Source: CAD feature listing. Evaluate the final solid. Frame: model axes, mm. Face numbers are marked on the shaded views. A direction names the side the tool comes from. Coordinates: 2 decimals unless noted, no trailing zeros. Write each loop counter-clockwise with the first axis right and the second up, starting at its lowest first coordinate (ties: lowest second). Pieces come first, ordered by that corner, then holes. Notation, with made-up numbers: (73, 73.25) - (99, 73.25) arc R27 cw to (99, 95.25) - close; hole circle Ø4 at (44.25, 31). An arc over 180 degrees is marked (long way). One line per question, with ' | ' between items.
from build123d import *

# Parameters (mm, degrees)
BOSS_EXTRUDE1_DEPTH = 7.5
FILLET1_R           = 6
FILLET2_R           = 4
BOSS_EXTRUDE2_DEPTH = 15
LPATTERN1_COUNT     = 6
LPATTERN1_PITCH     = 6
CUT_EXTRUDE1_DEPTH  = 26
CUT_EXTRUDE2_DEPTH  = 5
SKETCH5_R           = 1.5
CUT_EXTRUDE3_DEPTH  = 130.931165931
SKETCH6_R           = 1.75
BOSS_EXTRUDE3_DEPTH = 3
SKETCH7_R           = 1.25
CUT_EXTRUDE4_DEPTH  = 1
SKETCH8_R           = 1.25
CUT_EXTRUDE5_DEPTH  = 1
CUT_EXTRUDE6_DEPTH  = 1


with BuildPart() as part:
    # Sketch1 → Boss-Extrude1 (new, symmetric)
    with BuildSketch(Plane(origin=(0, 0, 0), x_dir=(0, 1, 0), z_dir=(0, 0, 1))):
        with BuildLine():
            Line((-12.93657624, 0), (-36.683093305, -3.478926169))
            Line((-36.683093305, -3.478926169), (-15.74375395, -70.273716889))
            Line((-15.74375395, -70.273716889), (-17.80717771, -70.273716889))
            Line((-17.80717771, -70.273716889), (-21.696997284, -79.486170616))
            Line((-21.696997284, -79.486170616), (-12.467013439, -88.640808687))
            Line((-12.467013439, -88.640808687), (-3.493010858, -117.267147567))
            Line((-3.493010858, -117.267147567), (-3.493010858, -124.267147567))
            Line((-3.493010858, -124.267147567), (6.506989142, -124.267147567))
            Line((6.506989142, -124.267147567), (6.506989142, -74.267147567))
            Line((6.506989142, -74.267147567), (12.638392495, -66.367407513))
            ThreePointArc((12.638392495, -66.367407513), (10.129821893, -59.756274968), (3.518689347, -62.26484557))
            Line((3.518689347, -62.26484557), (2.19282229, -70.273716889))
            Line((2.19282229, -70.273716889), (-2.80717771, -70.273716889))
            Line((-2.80717771, -70.273716889), (-12.93657624, 0))
        make_face()
    extrude(amount=BOSS_EXTRUDE1_DEPTH, both=True)

    # Fillet1
    fillet1_edges = [part.edges().sort_by_distance(p)[0] for p in [
        (3.478926169, -36.683093305, 0),
        (0, -12.93657624, 0),
    ]]
    fillet(fillet1_edges, radius=FILLET1_R)

    # Fillet2
    # the kernel refuses this fillet: 4 mm, written as the material it takes off along each edge
    with BuildSketch(Plane(origin=(124.267147567, -3.493010858, -17.5), x_dir=(0, 1, 0), z_dir=(0, 0, 1))) as fillet2_piece_1:
        with BuildLine():
            CenterArc((FILLET2_R, FILLET2_R), FILLET2_R, 180, 90)
            Line((0, FILLET2_R), (-FILLET2_R * 0.02, FILLET2_R))
            Line((-FILLET2_R * 0.02, FILLET2_R), (-FILLET2_R * 0.02, -FILLET2_R * 0.02))
            Line((-FILLET2_R * 0.02, -FILLET2_R * 0.02), (FILLET2_R, -FILLET2_R * 0.02))
            Line((FILLET2_R, -FILLET2_R * 0.02), (FILLET2_R, 0))
        make_face()
    extrude(amount=35, mode=Mode.SUBTRACT)
    with BuildSketch(Plane(origin=(70.273716889, -17.80717771, -14.005853421), x_dir=(0, 1, 0), z_dir=(0, 0, 1))) as fillet2_piece_2_section:
        with BuildLine():
            CenterArc((2.672717651, -3.953322774), FILLET2_R, 98.761599305, 58.347232051)
            Line((-1.012263839, -2.397394944), (-1.085963469, -2.366276387))
            Line((-1.085963469, -2.366276387), (-0.07369963, 0.031118557))
            Line((-0.07369963, 0.031118557), (0, 0.08))
            ThreePointArc((0, 0.08), (1.03171188, 0.08), (2.051237882, 0.079066455))
            Line((2.051237882, 0.079066455), (2.06342376, 0))
        make_face()
    fillet2_piece_2 = extrude(amount=28.011706842, mode=Mode.PRIVATE)
    fillet2_piece_2 = split(fillet2_piece_2, bisect_by=Plane(origin=(70.257081216, -15.748969027, 0), z_dir=(0.2991334193615799, -0.954211296003694, 0)), keep=Keep.TOP, mode=Mode.PRIVATE)
    add(fillet2_piece_2, mode=Mode.SUBTRACT)
    with BuildSketch(Plane(origin=(79.486170616, -21.696997284, -14.26109301), x_dir=(-0.9212453727262618, 0.3889819574613337, 0), z_dir=(0, 0, 1))) as fillet2_piece_3:
        with BuildLine():
            CenterArc((FILLET2_R * 0.676109301023, -FILLET2_R), FILLET2_R, 90, 68.125982867)
            Line((-FILLET2_R * 0.251896002422, -FILLET2_R * 0.627433017057), (-FILLET2_R * 0.270456108491, -FILLET2_R * 0.619981677398))
            Line((-FILLET2_R * 0.270456108491, -FILLET2_R * 0.619981677398), (-FILLET2_R * 0.0135221860205, FILLET2_R * 0.02))
            Line((-FILLET2_R * 0.0135221860205, FILLET2_R * 0.02), (FILLET2_R * 0.676109301023, FILLET2_R * 0.02))
            Line((FILLET2_R * 0.676109301023, FILLET2_R * 0.02), (FILLET2_R * 0.676109301023, 0))
        make_face()
    extrude(amount=28.52218602, mode=Mode.SUBTRACT)

    # Sketch2 → Boss-Extrude2 (add)
    with BuildSketch(Plane.XY.offset(7.5)):
        Polygon((119.267147567, 6.506989142), (121.267147567, 6.506989142), (119.267147567, 10.506989142), align=None)
        Polygon((117.267147567, 6.506989142), (119.267147567, 6.506989142), (119.267147567, 10.506989142), align=None)
    boss_extrude2 = extrude(amount=-BOSS_EXTRUDE2_DEPTH)

    # LPattern1: Boss-Extrude2 ×6
    with Locations(*[(-i * LPATTERN1_PITCH, 0, 0) for i in range(1, LPATTERN1_COUNT)]):
        add(boss_extrude2)

    # Sketch3 → Cut-Extrude1 (cut)
    with BuildSketch(Plane.XY.offset(7.5)):
        Polygon((118.41479062, 4.13462657), (86.532799982, 3.176685284), (86.532799982, -9.820815038), (116.995150337, -0.75112261), align=None)
    extrude(amount=-CUT_EXTRUDE1_DEPTH, mode=Mode.SUBTRACT)

    # Sketch4 → Cut-Extrude2 (cut)
    with BuildSketch(Plane(origin=(11.490191231, -36.652776175, 0), x_dir=(0.954211296003694, 0.2991334193615799, 0), z_dir=(0.29913341936157983, -0.9542112960036939, 0))):
        Polygon((85.852760577, 3.5), (85.852760577, -3.5), (106.852760577, -0.5), (106.852760577, 0.5), align=None)
    extrude(amount=-CUT_EXTRUDE2_DEPTH, mode=Mode.SUBTRACT)

    # Sketch5 → Cut-Extrude3 (cut, through all)
    with BuildSketch(Plane.XY.offset(7.5)):
        with Locations((8.395954367, -28.853750382)):
            Circle(SKETCH5_R)
    extrude(amount=-CUT_EXTRUDE3_DEPTH, mode=Mode.SUBTRACT)

    # Sketch6 → Boss-Extrude3 (add)
    with BuildSketch(Plane.XY.offset(7.5)):
        with Locations(Location((78.550648186, -16.960038516, 0), (0, 0, 180))):
            Circle(SKETCH6_R)
        with Locations(Location((64.316126541, 8.078540921, 0), (0, 0, 180))):
            Circle(SKETCH6_R)
    boss_extrude3 = extrude(amount=BOSS_EXTRUDE3_DEPTH)

    # Sketch7 → Cut-Extrude4 (cut)
    with BuildSketch(Plane.XY.offset(10.5)):
        with Locations((78.550648186, -16.960038516)):
            Circle(SKETCH7_R)
    cut_extrude4 = extrude(amount=-CUT_EXTRUDE4_DEPTH, mode=Mode.SUBTRACT)

    # Sketch8 → Cut-Extrude5 (cut)
    with BuildSketch(Plane.XY.offset(10.5)):
        with Locations((64.316126541, 8.078540921)):
            Circle(SKETCH8_R)
    cut_extrude5 = extrude(amount=-CUT_EXTRUDE5_DEPTH, mode=Mode.SUBTRACT)

    # Sketch9 → Cut-Extrude6 (cut)
    with BuildSketch(Plane.XY.offset(7.5)):
        with BuildLine():
            Line((15.753388713, -22.103953925), (62.646298586, -10.0457771))
            ThreePointArc((62.646298586, -10.0457771), (65.390728962, -11.667485959), (63.769020103, -14.411916335))
            Line((63.769020103, -14.411916335), (16.87611023, -26.470093159))
            ThreePointArc((16.87611023, -26.470093159), (14.131679854, -24.848384301), (15.753388713, -22.103953925))
        make_face()
    cut_extrude6 = extrude(amount=-CUT_EXTRUDE6_DEPTH, mode=Mode.SUBTRACT)

    # Mirror1: Boss-Extrude3, Cut-Extrude4, Cut-Extrude5, Cut-Extrude6 across plane
    add(boss_extrude3.mirror(Plane.XY))
    add(cut_extrude4.mirror(Plane.XY), mode=Mode.SUBTRACT)
    add(cut_extrude5.mirror(Plane.XY), mode=Mode.SUBTRACT)
    add(cut_extrude6.mirror(Plane.XY), mode=Mode.SUBTRACT)


solid = part.part
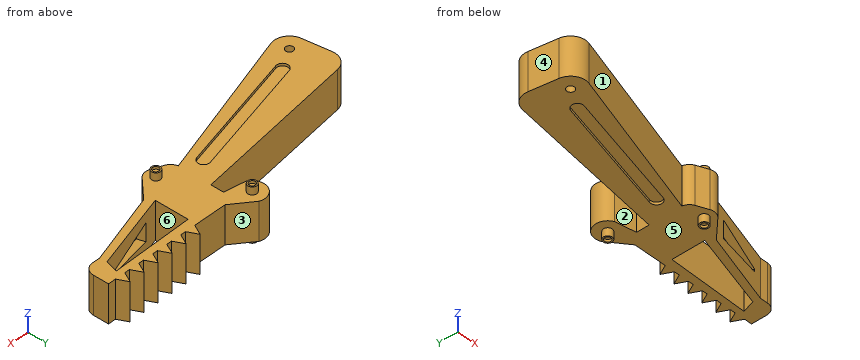
Item 1: Cut plane C-C on z = -4.75. State how many separate pieces and enclosed holes the cut face has, and give its area (3 significant figures).
Check sheet entries:
separate pieces: 1 | enclosed holes: 2 | area: 2,070 mm²
Item 2: Pin query (flat end, axial travel): pin 1 Ø5 at (x, z) = (14.5, -7.5) entering from +Y; pin 2 Ø3 at (x, z) = (24, -6) entering from -Y; pin 3 Ø2 at (x, y) = (55.5, -21.5) entering from +Z; pin 4 Ø2 at (x, y) = (21.5, -26) entering from +Z. Return the tip coordinate at first contact, or that it passes through.
Check sheet entries:
pin 1: y = -10.49 | pin 2: y = -30.72 | pin 3: through | pin 4: z = 7.5
Item 3: Cut plane D-D on x = 22. Return loops of the section in (y, z), and give its area (3 significant figures).
Check sheet entries:
outline: (-30.88, -7.5) - (-25.15, -7.5) - (-25.15, -6.5) - (-20.5, -6.5) - (-20.5, -7.5) - (-9.77, -7.5) - (-9.77, 7.5) - (-20.5, 7.5) - (-20.5, 6.5) - (-25.15, 6.5) - (-25.15, 7.5) - (-30.88, 7.5) - close | area: 307 mm²
Item 4: Ray query, line 1 along Z through (x, y) = (27.5, -22); line 2 along Z through (x, y) = (58, -7); line 3 along Y through (x, z) = (63, 3). Return the intervals inside material, ascending. Write a range as [from, to].
Check sheet entries:
line 1: [-6.5, 6.5] | line 2: [-7.5, 7.5] | line 3: [-18.02, -3.86], [3.4, 12.9]
Item 5: Mould query, pull axis X, two halves, no side actions, for the marked faces 4, 5 and 6. Classes: pulls with the +X half, pulls with the -X half, needs draft (parallel to the pull), parting line crosses it, or undercut.
Check sheet entries:
face 4: pulls with the -X half | face 5: needs draft | face 6: undercut
Item 6: Cut plane A-A on x = 68.5. Return loops of the section in (y, z).
Check sheet entries:
outline: (-16.3, -7.5) - (-3.06, -7.5) - (-3.06, 7.5) - (-16.3, 7.5) - close; (2.49, -7.5) - (10.98, -7.5) - (10.98, 7.5) - (2.49, 7.5) - close
Item 7: Access query for the marked faces 1, 2 and 3. Directions: +Z, -Z, +X, -X, +Y, -Y. A direction counts if a zero-diameter tool reaches every point of the face in a straight line with its end or side. Return the directions, or none.
Check sheet entries:
face 1: +Z, -Z, -Y | face 2: +Z, -Z, -X | face 3: +Z, -Z, +Y
Item 8: Cut plane B-B on x = 37.5. Return loops of the section in (y, z), and give its area (3 significant figures).
Check sheet entries:
outline: (-26.02, -7.5) - (-21.17, -7.5) - (-21.17, -6.5) - (-16.51, -6.5) - (-16.51, -7.5) - (-7.53, -7.5) - (-7.53, 7.5) - (-16.51, 7.5) - (-16.51, 6.5) - (-21.17, 6.5) - (-21.17, 7.5) - (-26.02, 7.5) - close | area: 268 mm²
